```python
from build123d import *

# Parameters (mm, degrees)
F0_W     = 62.291438
F0_H     = 41.213639
F0_W_2   = 97.35938
F0_H_2   = 154.007825
F0_R     = 7.65318
F0_W_3   = 52.04163
F0_H_3   = 45.17841
F1_DEPTH = 6.35


with BuildPart() as f1:
    # F0 (on Front) → F1 (new body)
    with BuildSketch(Plane.XZ):
        Polygon((151.493805, 99.992175), (-153.306195, 99.992175), (-153.458426, 43.937002), (-153.458426, -154.007825), (54.134425, -154.007825), (54.134425, 0), (151.493805, 0), align=None)
        with Locations((-17.055792, -54.690691)):
            Rectangle(F0_W, F0_H, mode=Mode.SUBTRACT)
        with Locations((102.814115, -77.003912)):
            Rectangle(F0_W_2, F0_H_2)
        with Locations((130.116299, -90.2858)):
            Circle(F0_R, mode=Mode.SUBTRACT)
        with Locations((98.637318, -54.690691)):
            Rectangle(F0_W_3, F0_H_3, mode=Mode.SUBTRACT)
    extrude(amount=F1_DEPTH)


solid = f1.part
```
Geometry: final body of the model. Coordinates: model frame, mm. A direction names the side the tool comes from. Coordinates: 2 decimals unless noted, no trailing zeros. Write each loop counter-clockwise with the first axis right and the second up, starting at its lowest first coordinate (ties: lowest second). Pieces come first, ordered by that corner, then holes. Notation, with made-up numbers: M 34.5,9 L 41.5,9 A27 ccw 41.5,37 Z; hole C 31.5,23 d5. An arc over 180 degrees is marked long. Answer as CSV lines item,"result". Start each with the question number.
Q1. Reachability of faces 4 (the flat face through (98, -3, -32.101)), 5 (the flat face through (1, -3, 99.992)) from +Z, -Z, +X, -X, +Y, -Y: full face, straight path, thin tool, end or side. Return the list, or none.
Q2. Cut plane C-C on y = -1. Return the cut outline in (x, z).
Q3. Cut plane A-A on x = -14. Return the cut outline in (y, z).
Q4. Cut plane B-B on x = 80. Return the cut outline in (y, z), then the cut area to 3 significant figures.
Q5. Mould query, pull axis Z, two halves, no side actions, for faces 1 (the flat face through (-3, 0, -25)), 2 (the flat face through (102, -3, -154.008)), 3 (the flat face through (124.658, -3, -55)). Classes: released by +Z, released by -Z, zero draft, split by the parting line, or undercut.
Q6. Line query: line 1 (X direction, y = -1.5, z = -65); line 2 (Z direction, x = 1, y = -2.5); line 3 (X direction, y = -4, z = -77). Output: solid intervals per line, ascending. Write a range as from..to.
Q7. Pin query (flat end, axial travel): P1, Ø9, axis at x = 130.12, z = -90.29, coming from the -Y side. Return the tip coordinate at first contact, or that it passes through.
Findings below:
1,face 4,"+Y, -Y"
1,face 5,"+Z, +X, -X, +Y, -Y"
2,outline,"M -153.46,-154.01 L 151.49,-154.01 L 151.49,99.99 L -153.31,99.99 L -153.46,43.94 Z; hole M -48.2,-75.3 L 14.09,-75.3 L 14.09,-34.08 L -48.2,-34.08 Z; hole M 72.62,-77.28 L 124.66,-77.28 L 124.66,-32.1 L 72.62,-32.1 Z; hole C 130.12,-90.29 d15.31"
3,outline,"M -6.35,-154.01 L 0,-154.01 L 0,-75.3 L -6.35,-75.3 Z; M -6.35,-34.08 L 0,-34.08 L 0,99.99 L -6.35,99.99 Z"
4,outline,"M -6.35,-154.01 L 0,-154.01 L 0,-77.28 L -6.35,-77.28 Z; M -6.35,-32.1 L 0,-32.1 L 0,99.99 L -6.35,99.99 Z"
4,area,"1,330 mm2"
5,face 1,"zero draft"
5,face 2,"released by -Z"
5,face 3,"undercut"
6,line 1,"x = -153.46..-48.2, 14.09..72.62, 124.66..151.49"
6,line 2,"z = -154.01..-75.3, -34.08..99.99"
6,line 3,"x = -153.46..72.62, 124.66..151.49"
7,P1,"passes through"
